```python
from build123d import *

# Parameters (mm, degrees)
SKETCH1_R           = 24
SKETCH1_R_2         = 1.1
BOSS_EXTRUDE1_DEPTH = 1.6
FILLET1_R           = 1
SKETCH2_R           = 2.5
CUT_EXTRUDE1_DEPTH  = 34.978816931


with BuildPart() as part:
    # Sketch1 → Boss-Extrude1 (new body)
    with BuildSketch(Plane(origin=(0, 0, 0), x_dir=(1, 0, 0), z_dir=(0, 1, 0))):
        with Locations(Location((0, 0, 0), (0, 0, 270))):
            Circle(SKETCH1_R)
        with BuildLine():
            Line((-7.463736271, -16.927570436), (0, -4))
            Line((0, -4), (7.463736271, -16.927570436))
            ThreePointArc((7.463736271, -16.927570436), (0, -18.5), (-7.463736271, -16.927570436))
        make_face(mode=Mode.SUBTRACT)
        with BuildLine():
            Line((10.927837886, -14.927570436), (3.464101615, -2))
            Line((3.464101615, -2), (18.391574158, -2))
            ThreePointArc((18.391574158, -2), (16.02146997, -9.25), (10.927837886, -14.927570436))
        make_face(mode=Mode.SUBTRACT)
        with BuildLine():
            Line((18.391574158, 2), (3.464101615, 2))
            Line((3.464101615, 2), (10.927837886, 14.927570436))
            ThreePointArc((10.927837886, 14.927570436), (16.02146997, 9.25), (18.391574158, 2))
        make_face(mode=Mode.SUBTRACT)
        with BuildLine():
            Line((7.463736271, 16.927570436), (0, 4))
            Line((0, 4), (-7.463736271, 16.927570436))
            ThreePointArc((-7.463736271, 16.927570436), (0, 18.5), (7.463736271, 16.927570436))
        make_face(mode=Mode.SUBTRACT)
        with BuildLine():
            Line((-10.927837886, 14.927570436), (-3.464101615, 2))
            Line((-3.464101615, 2), (-18.391574158, 2))
            ThreePointArc((-18.391574158, 2), (-16.02146997, 9.25), (-10.927837886, 14.927570436))
        make_face(mode=Mode.SUBTRACT)
        with BuildLine():
            Line((-18.391574158, -2), (-3.464101615, -2))
            Line((-3.464101615, -2), (-10.927837886, -14.927570436))
            ThreePointArc((-10.927837886, -14.927570436), (-16.02146997, -9.25), (-18.391574158, -2))
        make_face(mode=Mode.SUBTRACT)
        with Locations(Location((-10.60675, -18.371429903, 0), (0, 0, 270))):
            Circle(SKETCH1_R_2, mode=Mode.SUBTRACT)
        with Locations(Location((-21.2135, 0, 0), (0, 0, 270))):
            Circle(SKETCH1_R_2, mode=Mode.SUBTRACT)
        with Locations(Location((10.60675, -18.371429903, 0), (0, 0, 270))):
            Circle(SKETCH1_R_2, mode=Mode.SUBTRACT)
        with Locations(Location((21.2135, 0, 0), (0, 0, 270))):
            Circle(SKETCH1_R_2, mode=Mode.SUBTRACT)
        with Locations(Location((-10.60675, 18.371429903, 0), (0, 0, 270))):
            Circle(SKETCH1_R_2, mode=Mode.SUBTRACT)
        with Locations(Location((10.60675, 18.371429903, 0), (0, 0, 270))):
            Circle(SKETCH1_R_2, mode=Mode.SUBTRACT)
    extrude(amount=BOSS_EXTRUDE1_DEPTH)

    # Fillet1
    fillet1_edges = [part.edges().sort_by_distance(p)[0] for p in [
        (-3.464101615, 0.8, 2),
        (-18.391574158, 0.8, 2),
        (-10.927837886, 0.8, 14.927570436),
        (-18.391574158, 0.8, -2),
        (-3.464101615, 0.8, -2),
        (-10.927837886, 0.8, -14.927570436),
        (-7.463736271, 0.8, 16.927570436),
        (7.463736271, 0.8, 16.927570436),
        (0, 0.8, 4),
        (10.927837886, 0.8, 14.927570436),
        (18.391574158, 0.8, 2),
        (3.464101615, 0.8, 2),
        (18.391574158, 0.8, -2),
        (10.927837886, 0.8, -14.927570436),
        (3.464101615, 0.8, -2),
        (7.463736271, 0.8, -16.927570436),
        (-7.463736271, 0.8, -16.927570436),
        (0, 0.8, -4),
    ]]
    fillet(fillet1_edges, radius=FILLET1_R)

    # Sketch2 → Cut-Extrude1 (cut, through all)
    with BuildSketch(Plane(origin=(0, 1.6, 0), x_dir=(1, 0, 0), z_dir=(0, 1, 0))):
        with Locations(Location((0, 0, 0), (0, 0, 270))):
            Circle(SKETCH2_R)
    extrude(amount=-CUT_EXTRUDE1_DEPTH, mode=Mode.SUBTRACT)


solid = part.part
```
Check sheet for the modelled part. Datum: model origin and axes. Units: mm. Give positions to 0.01 mm unless a question says otherwise; leave off trailing zeros. Order: outer loops, then holes, each group sorted by start corner. A loop starts at its lowest first (then second) coordinate and runs counter-clockwise, first axis right, second up. Notation, with made-up numbers: (74.25, 53) -> (111.25, 53) arc R25 ccw to (111.25, 82) -> close; hole circle Ø8 at (-38, 46.25). An arc over 180 degrees is marked (long way). Use CSV: the item, a comma, the result in double quotes. Start each with the question number.
1) Sectioned sample at C-C, the plane y = 0.3. Give the number of separate pieces and of enclosed holes in the cut face, plus the area to 3 significant figures.
2) Sectioned sample at A-A, the plane x = 0. Record the boundary of the cut face in (y, z).
3) Material ranges on line 1 (X direction, y = 0.55, z = 0); line 2 (X direction, y = 0.2, z = -12.5); line 3 (X direction, y = 1.4, z = -4.5), recorded low to high. Write a range as from..to.
4) Mould release check, pull along Z, two halves, no side actions. Record for faces 1 (the face through (11.35, 0.79, -19.18)), 2 (the face through (-3.92, 0.79, 10.79)), 3 (the face through (7.21, 0.79, 22.89)): released by +Z, released by -Z, zero draft, split by the parting line, or undercut.
5) Go/stop test with flat-tipped pins: P1, Ø0.8, axis at x = 11.5, y = 1, coming from the +Z side; P2, Ø3.5, axis at x = 10.61, z = 18.37, coming from the -Y side; P3, Ø0.5, axis at x = 12, y = 1, coming from the -Z side; P4, Ø1.3, axis at x = -21.21, z = 0, coming from the +Y side. Record where each tip stops, or that it passes through.
6) Sectioned sample at B-B, the plane z = 0. Record the boundary of the cut face in (x, y), plus the area to 3 significant figures.
Recorded:
1,separate pieces,"1"
1,enclosed holes,"13"
1,area,"1,100 mm2"
2,outline,"(0, -24) -> (1.6, -24) -> (1.6, -18.5) -> (0, -18.5) -> close; (0, -5) -> (1.6, -5) -> (1.6, -2.5) -> (0, -2.5) -> close; (0, 2.5) -> (1.6, 2.5) -> (1.6, 5) -> (0, 5) -> close; (0, 18.5) -> (1.6, 18.5) -> (1.6, 24) -> (0, 24) -> close"
3,line 1,"-24..-22.31, -20.11..-2.5, 2.5..20.11, 22.31..24"
3,line 2,"-20.49..-13.64, -9.53..-4.91, 4.91..9.53, 13.64..20.49"
3,line 3,"-23.57..-17.94, -4.91..4.91, 17.94..23.57"
4,face 1,"undercut"
4,face 2,"undercut"
4,face 3,"split by the parting line"
5,P1,"z = 21.28"
5,P2,"y = 0"
5,P3,"z = -20.93"
5,P4,"through"
6,outline,"(-24, 0) -> (-22.31, 0) -> (-22.31, 1.6) -> (-24, 1.6) -> close; (-20.11, 0) -> (-2.5, 0) -> (-2.5, 1.6) -> (-20.11, 1.6) -> close; (2.5, 0) -> (20.11, 0) -> (20.11, 1.6) -> (2.5, 1.6) -> close; (22.31, 0) -> (24, 0) -> (24, 1.6) -> (22.31, 1.6) -> close"
6,area,"61.8 mm2"
